```python
from build123d import *

# Parameters (mm, degrees)
F0_W     = 34
F0_H     = 31
F1_DEPTH = 9
F2_DEPTH = 6.5
F3_START = 6
F0_W_2   = 2.5
F0_H_2   = 3
F3_DEPTH = 3
F4_START = 6
F0_R     = 2
F4_DEPTH = 12
F5_SIZE  = 0.75
F6_SIZE  = 0.75


with BuildPart() as f1:
    # F0 (on Top) → F1 (new body)
    with BuildSketch(Plane.XY):
        with BuildLine():
            Line((-4.5, 17.5), (-17, 17.5))
            Line((-17, 17.5), (-17, -17.5))
            Line((-17, -17.5), (-4.5, -17.5))
            Line((-4.5, -17.5), (-2.0348525745, -17.5))
            ThreePointArc((-2.0348525745, -17.5), (0, -16.875), (2.0348525745, -17.5))
            Line((2.0348525745, -17.5), (4.5, -17.5))
            Line((4.5, -17.5), (21, -17.5))
            Line((21, -17.5), (21, 17.5))
            Line((21, 17.5), (4.5, 17.5))
            Line((4.5, 17.5), (2.0348525745, 17.5))
            ThreePointArc((2.0348525745, 17.5), (0, 16.875), (-2.0348525745, 17.5))
            Line((-2.0348525745, 17.5), (-4.5, 17.5))
        make_face()
        with Locations((2, 0)):
            Rectangle(F0_W, F0_H, mode=Mode.SUBTRACT)
        with BuildLine():
            Line((-4.5, 20.5), (-4.5, 17.5))
            Line((-4.5, 17.5), (-2.0348525745, 17.5))
            ThreePointArc((-2.0348525745, 17.5), (-3.2028866342, 18.8023126882), (-3.625, 20.5))
            Line((-3.625, 20.5), (-4.5, 20.5))
        make_face()
        with BuildLine():
            ThreePointArc((4.5, 20.5), (0, 25), (-4.5, 20.5))
            Line((-4.5, 20.5), (-3.625, 20.5))
            ThreePointArc((-3.625, 20.5), (0, 24.125), (3.625, 20.5))
            Line((3.625, 20.5), (4.5, 20.5))
        make_face()
        with BuildLine():
            ThreePointArc((3.625, 20.5), (3.2028866342, 18.8023126882), (2.0348525745, 17.5))
            Line((2.0348525745, 17.5), (4.5, 17.5))
            Line((4.5, 17.5), (4.5, 20.5))
            Line((4.5, 20.5), (3.625, 20.5))
        make_face()
        with BuildLine():
            Line((4.5, -17.5), (2.0348525745, -17.5))
            ThreePointArc((2.0348525745, -17.5), (3.2028866342, -18.8023126882), (3.625, -20.5))
            Line((3.625, -20.5), (4.5, -20.5))
            Line((4.5, -20.5), (4.5, -17.5))
        make_face()
        with BuildLine():
            Line((-2.0348525745, -17.5), (-4.5, -17.5))
            Line((-4.5, -17.5), (-4.5, -20.5))
            Line((-4.5, -20.5), (-3.625, -20.5))
            ThreePointArc((-3.625, -20.5), (-3.2028866342, -18.8023126882), (-2.0348525745, -17.5))
        make_face()
        with BuildLine():
            Line((-3.625, -20.5), (-4.5, -20.5))
            ThreePointArc((-4.5, -20.5), (0, -25), (4.5, -20.5))
            Line((4.5, -20.5), (3.625, -20.5))
            ThreePointArc((3.625, -20.5), (0, -24.125), (-3.625, -20.5))
        make_face()
    extrude(amount=F1_DEPTH)

    # F0 (on Top) → F2 (join)
    with BuildSketch(Plane.XY):
        with BuildLine():
            ThreePointArc((-3.625, 20.5), (-3.2028866342, 18.8023126882), (-2.0348525745, 17.5))
            Line((-2.0348525745, 17.5), (2.0348525745, 17.5))
            ThreePointArc((2.0348525745, 17.5), (3.2028866342, 18.8023126882), (3.625, 20.5))
            Line((3.625, 20.5), (1.875, 20.5))
            ThreePointArc((1.875, 20.5), (0, 18.625), (-1.875, 20.5))
            Line((-1.875, 20.5), (-3.625, 20.5))
        make_face()
        with BuildLine():
            Line((2.0348525745, 17.5), (-2.0348525745, 17.5))
            ThreePointArc((-2.0348525745, 17.5), (0, 16.875), (2.0348525745, 17.5))
        make_face()
        with BuildLine():
            ThreePointArc((3.625, 20.5), (0, 24.125), (-3.625, 20.5))
            Line((-3.625, 20.5), (-1.875, 20.5))
            ThreePointArc((-1.875, 20.5), (0, 22.375), (1.875, 20.5))
            Line((1.875, 20.5), (3.625, 20.5))
        make_face()
        with BuildLine():
            Line((2.0348525745, -17.5), (-2.0348525745, -17.5))
            ThreePointArc((-2.0348525745, -17.5), (-3.2028866342, -18.8023126882), (-3.625, -20.5))
            Line((-3.625, -20.5), (-1.875, -20.5))
            ThreePointArc((-1.875, -20.5), (0, -18.625), (1.875, -20.5))
            Line((1.875, -20.5), (3.625, -20.5))
            ThreePointArc((3.625, -20.5), (3.2028866342, -18.8023126882), (2.0348525745, -17.5))
        make_face()
        with BuildLine():
            ThreePointArc((2.0348525745, -17.5), (0, -16.875), (-2.0348525745, -17.5))
            Line((-2.0348525745, -17.5), (2.0348525745, -17.5))
        make_face()
        with BuildLine():
            Line((-1.875, -20.5), (-3.625, -20.5))
            ThreePointArc((-3.625, -20.5), (0, -24.125), (3.625, -20.5))
            Line((3.625, -20.5), (1.875, -20.5))
            ThreePointArc((1.875, -20.5), (0, -22.375), (-1.875, -20.5))
        make_face()
    extrude(amount=F2_DEPTH)

    # F0 (on Top) → F3 (join)
    with BuildSketch(Plane.XY.offset(F3_START)):
        with Locations((2, 0)):
            Rectangle(F0_W, F0_H)
        with BuildLine():
            ThreePointArc((1.25, 4.8412291828), (3.5355339059, 3.5355339059), (4.8412291828, 1.25))
            Line((4.8412291828, 1.25), (11.5, 1.25))
            Line((11.5, 1.25), (11.5, 4.25))
            Line((11.5, 4.25), (14, 4.25))
            Line((14, 4.25), (14, 1.25))
            Line((14, 1.25), (14, -1.25))
            Line((14, -1.25), (14, -4.25))
            Line((14, -4.25), (11.5, -4.25))
            Line((11.5, -4.25), (11.5, -1.25))
            Line((11.5, -1.25), (4.8412291828, -1.25))
            ThreePointArc((4.8412291828, -1.25), (3.5355339059, -3.5355339059), (1.25, -4.8412291828))
            Line((1.25, -4.8412291828), (1.25, -8))
            Line((1.25, -8), (15, -8))
            Line((15, -8), (15, -10.5))
            Line((15, -10.5), (-11, -10.5))
            Line((-11, -10.5), (-11, -8))
            Line((-11, -8), (-1.25, -8))
            Line((-1.25, -8), (-1.25, -4.8412291828))
            ThreePointArc((-1.25, -4.8412291828), (-3.5355339059, -3.5355339059), (-4.8412291828, -1.25))
            Line((-4.8412291828, -1.25), (-7.5, -1.25))
            Line((-7.5, -1.25), (-7.5, -4.25))
            Line((-7.5, -4.25), (-10, -4.25))
            Line((-10, -4.25), (-10, -1.25))
            Line((-10, -1.25), (-10, 1.25))
            Line((-10, 1.25), (-10, 4.25))
            Line((-10, 4.25), (-7.5, 4.25))
            Line((-7.5, 4.25), (-7.5, 1.25))
            Line((-7.5, 1.25), (-4.8412291828, 1.25))
            ThreePointArc((-4.8412291828, 1.25), (-3.5355339059, 3.5355339059), (-1.25, 4.8412291828))
            Line((-1.25, 4.8412291828), (-1.25, 8))
            Line((-1.25, 8), (-11, 8))
            Line((-11, 8), (-11, 10.5))
            Line((-11, 10.5), (15, 10.5))
            Line((15, 10.5), (15, 8))
            Line((15, 8), (1.25, 8))
            Line((1.25, 8), (1.25, 4.8412291828))
        make_face(mode=Mode.SUBTRACT)
        with Locations((-8.75, 2.75)):
            Rectangle(F0_W_2, F0_H_2)
        with BuildLine():
            ThreePointArc((-4.8412291828, -1.25), (-5, 0), (-4.8412291828, 1.25))
            Line((-4.8412291828, 1.25), (-7.5, 1.25))
            Line((-7.5, 1.25), (-10, 1.25))
            Line((-10, 1.25), (-10, -1.25))
            Line((-10, -1.25), (-7.5, -1.25))
            Line((-7.5, -1.25), (-4.8412291828, -1.25))
        make_face()
        with Locations((-8.75, -2.75)):
            Rectangle(F0_W_2, F0_H_2)
        Polygon((15, -8), (1.25, -8), (-1.25, -8), (-11, -8), (-11, -10.5), (15, -10.5), align=None)
        with BuildLine():
            Line((1.25, -8), (1.25, -4.8412291828))
            ThreePointArc((1.25, -4.8412291828), (0, -5), (-1.25, -4.8412291828))
            Line((-1.25, -4.8412291828), (-1.25, -8))
            Line((-1.25, -8), (1.25, -8))
        make_face()
        with Locations((12.75, -2.75)):
            Rectangle(F0_W_2, F0_H_2)
        with Locations((12.75, 2.75)):
            Rectangle(F0_W_2, F0_H_2)
        with BuildLine():
            ThreePointArc((4.8412291828, 1.25), (4.9601484813, 0.6300214624), (5, 0))
            ThreePointArc((5, 0), (4.9601484813, -0.6300214624), (4.8412291828, -1.25))
            Line((4.8412291828, -1.25), (11.5, -1.25))
            Line((11.5, -1.25), (14, -1.25))
            Line((14, -1.25), (14, 1.25))
            Line((14, 1.25), (11.5, 1.25))
            Line((11.5, 1.25), (4.8412291828, 1.25))
        make_face()
        Polygon((-1.25, 8), (1.25, 8), (15, 8), (15, 10.5), (-11, 10.5), (-11, 8), align=None)
        with BuildLine():
            ThreePointArc((-1.25, 4.8412291828), (0, 5), (1.25, 4.8412291828))
            Line((1.25, 4.8412291828), (1.25, 8))
            Line((1.25, 8), (-1.25, 8))
            Line((-1.25, 8), (-1.25, 4.8412291828))
        make_face()
    extrude(amount=F3_DEPTH)

    # F0 (on Top) → F4 (join)
    with BuildSketch(Plane.XY.offset(F4_START)):
        with BuildLine():
            Line((2.5, 1.25), (4.8412291828, 1.25))
            ThreePointArc((4.8412291828, 1.25), (3.5355339059, 3.5355339059), (1.25, 4.8412291828))
            Line((1.25, 4.8412291828), (1.25, 2.5))
            Line((1.25, 2.5), (-1.25, 2.5))
            Line((-1.25, 2.5), (-1.25, 4.8412291828))
            ThreePointArc((-1.25, 4.8412291828), (-3.5355339059, 3.5355339059), (-4.8412291828, 1.25))
            Line((-4.8412291828, 1.25), (-2.5, 1.25))
            Line((-2.5, 1.25), (-2.5, -1.25))
            Line((-2.5, -1.25), (-4.8412291828, -1.25))
            ThreePointArc((-4.8412291828, -1.25), (-3.5355339059, -3.5355339059), (-1.25, -4.8412291828))
            Line((-1.25, -4.8412291828), (-1.25, -2.5))
            Line((-1.25, -2.5), (1.25, -2.5))
            Line((1.25, -2.5), (1.25, -4.8412291828))
            ThreePointArc((1.25, -4.8412291828), (3.5355339059, -3.5355339059), (4.8412291828, -1.25))
            Line((4.8412291828, -1.25), (2.5, -1.25))
            Line((2.5, -1.25), (2.5, 1.25))
        make_face()
        Circle(F0_R, mode=Mode.SUBTRACT)
        with BuildLine():
            Line((-2.5, 1.25), (-4.8412291828, 1.25))
            ThreePointArc((-4.8412291828, 1.25), (-5, 0), (-4.8412291828, -1.25))
            Line((-4.8412291828, -1.25), (-2.5, -1.25))
            Line((-2.5, -1.25), (-2.5, 1.25))
        make_face()
        with BuildLine():
            ThreePointArc((-1.25, -4.8412291828), (0, -5), (1.25, -4.8412291828))
            Line((1.25, -4.8412291828), (1.25, -2.5))
            Line((1.25, -2.5), (-1.25, -2.5))
            Line((-1.25, -2.5), (-1.25, -4.8412291828))
        make_face()
        with BuildLine():
            ThreePointArc((4.8412291828, -1.25), (4.9601484813, -0.6300214624), (5, 0))
            ThreePointArc((5, 0), (4.9601484813, 0.6300214624), (4.8412291828, 1.25))
            Line((4.8412291828, 1.25), (2.5, 1.25))
            Line((2.5, 1.25), (2.5, -1.25))
            Line((2.5, -1.25), (4.8412291828, -1.25))
        make_face()
        with BuildLine():
            Line((1.25, 2.5), (1.25, 4.8412291828))
            ThreePointArc((1.25, 4.8412291828), (0, 5), (-1.25, 4.8412291828))
            Line((-1.25, 4.8412291828), (-1.25, 2.5))
            Line((-1.25, 2.5), (1.25, 2.5))
        make_face()
    extrude(amount=F4_DEPTH)

    # F5
    f5_edges = [f1.edges().sort_by_distance(p)[0] for p in [
        (-1.25, -4.841229, 18),
    ]]
    chamfer(f5_edges, length=F5_SIZE)

    # F6
    f6_edges = [f1.edges().sort_by_distance(p)[0] for p in [
        (1.875, 20.5, 0),
    ]]
    chamfer(f6_edges, length=F6_SIZE)


solid = f1.part
```
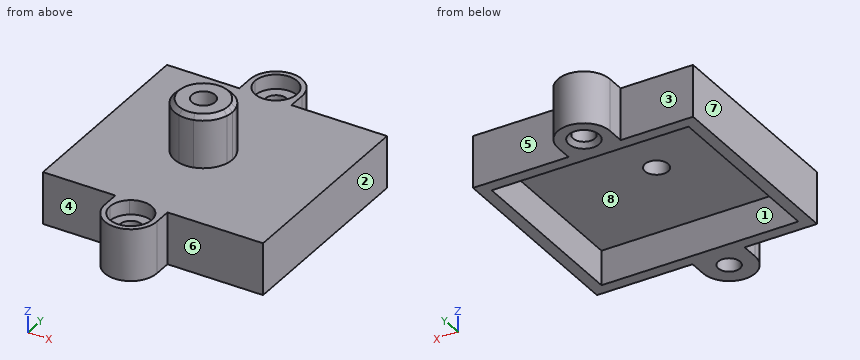
Geometry check sheet. Reference: the model listing, model coordinates, mm. Face numbers are marked on the shaded views. A direction names the side the tool comes from. Give positions to 0.01 mm unless a question says otherwise; leave off trailing zeros. Loops run counter-clockwise (first coordinate to the right, second up) from the corner with the lowest first, then second, coordinate; pieces in that order, holes last. Notation, with made-up numbers: (46, 32.25) - (102, 32.25) arc R18 cw to (102, 61.25) - close; hole circle Ø7 at (4, 45). An arc over 180 degrees is marked (long way). Use CSV: the item, a comma, the result in double quotes. Start each with the question number.
Q1. Scan lines: probe 1 along Y at (x, z) = (0, 3.25) (3 decimals); probe 2 along Y at (x, z) = (-7, 1.5); probe 3 along Y at (x, z) = (0, 13.75). Record each from-to range of solid material in increasing order. Write a range as from..to.
Q2. Section check B-B, the plane x = 0. Count the separate pieces of the cut face and the enclosed holes in it, and give its area (3 significant figures).
Q3. Go/stop test with flat-tipped pins: pin 1 Ø7 at (x, z) = (13.5, 3) entering from +Y; pin 2 Ø10 at (x, z) = (17, 16) entering from +Y; pin 3 Ø6 at (x, y) = (-0.5, -19.5) entering from +Z; pin 4 Ø6 at (x, z) = (13.5, 9.5) entering from -Y. Record where each tip stops, or that it passes through.
Q4. Section check C-C, the plane x = 16. Record the cut outline in (y, z).
Q5. Access from +Z, -Z, +X, -X, +Y, -Y to the whole of each face (thin tool, end or side, straight path). Record for the marked faces 1, 2, 3, 4 and 5.
Q6. Release check for a two-part mould opening along Y. For the marked faces 6, 7 and 8 record: +Y half, -Y half, draft (parallel to the pull), parting line (faces both ways), or undercut.
Q7. Section check A-A, the plane z = 3.75. Record the cut outline in (x, y) (3 decimals), and give its area (3 significant figures).
Findings below:
1,probe 1,"y = -25..-22.375, -18.625..-15.5, 15.5..18.625, 22.375..25"
1,probe 2,"y = -17.5..-15.5, 15.5..17.5"
1,probe 3,"y = -5..-2, 2..5"
2,separate pieces,"4"
2,enclosed holes,"0"
2,area,"220 mm^2"
3,pin 1,"stops at y = 17.5"
3,pin 2,"passes through"
3,pin 3,"stops at z = 9"
3,pin 4,"stops at y = -17.5"
4,outline,"(-17.5, 0) - (-15.5, 0) - (-15.5, 6) - (15.5, 6) - (15.5, 0) - (17.5, 0) - (17.5, 9) - (-17.5, 9) - close"
5,face 1,"-Z"
5,face 2,"+Z, -Z, +X, +Y, -Y"
5,face 3,"+Z, -Z, -X, +Y"
5,face 4,"+Z, -Z, -X, -Y"
5,face 5,"+Z, -Z, +X, +Y"
6,face 6,"-Y half"
6,face 7,"draft"
6,face 8,"undercut"
7,outline,"(-17, -17.5) - (-4.5, -17.5) - (-4.5, -20.5) arc R4.5 ccw to (4.5, -20.5) - (4.5, -17.5) - (21, -17.5) - (21, 17.5) - (4.5, 17.5) - (4.5, 20.5) arc R4.5 ccw to (-4.5, 20.5) - (-4.5, 17.5) - (-17, 17.5) - close; hole (-15, -15.5) - (19, -15.5) - (19, 15.5) - (-15, 15.5) - close; hole circle Ø3.75 at (0, -20.5); hole circle Ø3.75 at (0, 20.5)"
7,area,"372 mm^2"
